Job drawing, mm, ordinate dimensions from the low corner. One solid piece. A direction names the side the tool comes from. Round coordinates to 2 decimals unless told otherwise and drop trailing zeros. Write each loop counter-clockwise with the first axis right and the second up, starting at its lowest first coordinate (ties: lowest second). Pieces come first, ordered by that corner, then holes. Notation, with made-up numbers: M -12.5,17.25 L 1.5,17.25 A14 cw 1.5,23.25 Z; hole C -23,55 d2. An arc over 180 degrees is marked long. Answer as a JSON object with one key per item and string values. Group by question number.
1. Drop flat-ended pins along their axis: pin 1 (3 mm diameter, centred on y = 5.5, z = 15, fed in from +X); pin 2 (4 mm diameter, centred on y = 1.5, z = 27.5, fed in from +X); pin 3 (1 mm diameter, centred on y = 5, z = 24, fed in from -X). Give the stop position or say it passes through.
2. Band-saw the part on C-C, the plane y = 7.5. Write the cut outline in (x, z), plus the area to 3 significant figures.
3. Band-saw the part on D-D, the plane x = 2.25. Write the cut outline in (y, z), plus the area to 3 significant figures.
4. Band-saw the part on B-B, the plane z = 19.5. Write the cut outline in (x, y).
5. Drill centre lines: line 1 (Z direction, x = 1.5, y = 3.25); line 2 (Z direction, x = 9.25, y = 2.75); line 3 (X direction, y = 9.5, z = 27). Where is each one in solid material? Low to high. Write a range as from..to.
6. Which spindle directions (+Z, -Z, +X, -X, +Y, -Y) get a long thin tool onto all of the face, cutting with end or side? Do the marked faces 1, 2, 3, 4 and 5. Say none if no direction does.
7. Band-saw the part on A-A, the plane x = 7. Write the cut outline in (y, z).
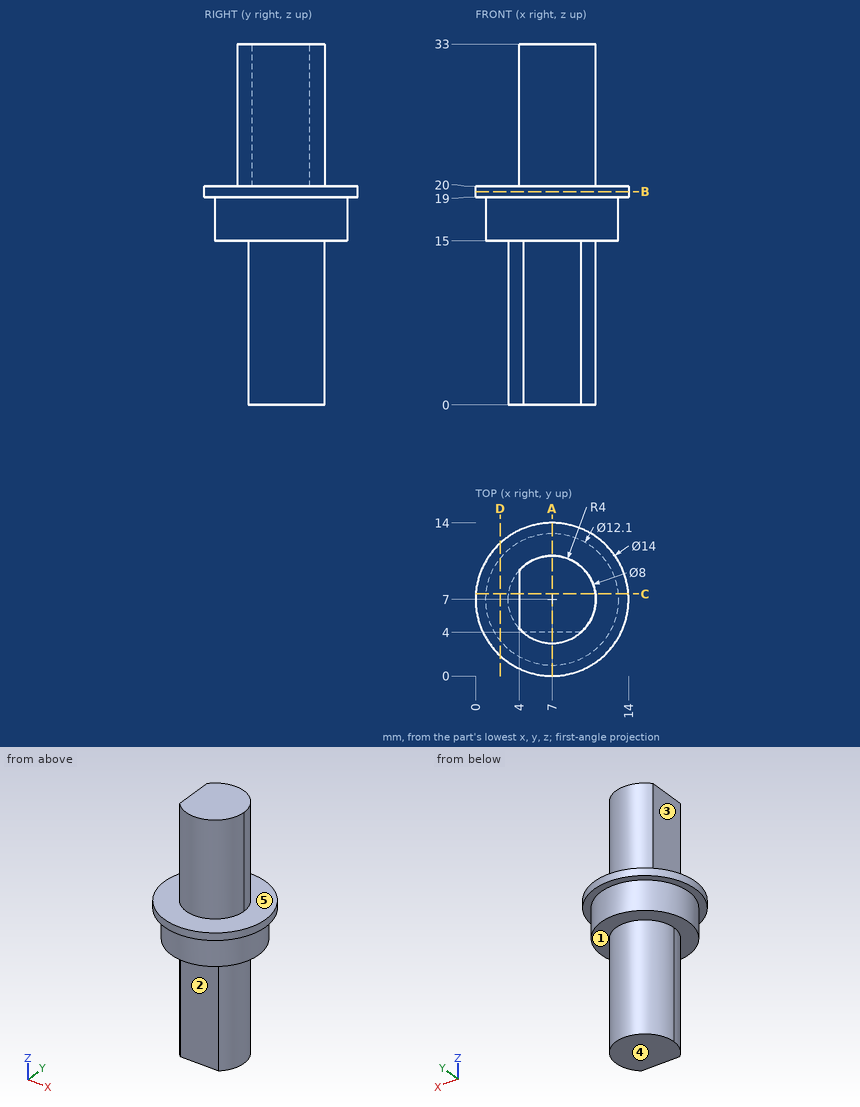
Worked answers:
{
 "1": {"pin 1": "stops at x = 13.05", "pin 2": "stops at x = 8.94", "pin 3": "stops at x = 4"},
 "2": {"outline": "M 0.02,19 L 0.97,19 L 0.97,15 L 3.03,15 L 3.03,0 L 10.97,0 L 10.97,15 L 13.03,15 L 13.03,19 L 13.98,19 L 13.98,20 L 10.97,20 L 10.97,33 L 4,33 L 4,20 L 0.02,20 Z", "area": "272 mm^2"},
 "3": {"outline": "M 1.86,19 L 3.25,19 L 3.25,15 L 10.75,15 L 10.75,19 L 12.14,19 L 12.14,20 L 1.86,20 Z", "area": "40.3 mm^2"},
 "4": {"outline": "C 7,7 d14"},
 "5": {"line 1": "z = 19..20", "line 2": "z = 15..20", "line 3": "x = 4..10.12"},
 "6": {"face 1": "-Z", "face 2": "-Z, +X, -X, -Y", "face 3": "+Z, -X, +Y, -Y", "face 4": "-Z, +X, -X, +Y, -Y", "face 5": "+Z"},
 "7": {"outline": "M 0,19 L 0.95,19 L 0.95,15 L 4,15 L 4,0 L 11,0 L 11,15 L 13.05,15 L 13.05,19 L 14,19 L 14,20 L 11,20 L 11,33 L 3,33 L 3,20 L 0,20 Z"}
}
